Autodesk Inventor part; units mm, degrees
ref_plane "Arbeitsebene1" through (0, 0, 4) normal (0, 0, 1) x (1, 0, 0)
ref_plane "YZ Plane" through (0, 0, 0) normal (1, 0, 0) x (0, 1, 0)
ref_plane "XZ Plane" through (0, 0, 0) normal (0, 1, 0) x (-1, 0, 0)
sketch "Skizze1" plane through (0, 0, 0) normal (0, 0, 1) x (1, 0, 0)
  line L0 (-27, -12) -> (27, -12)
  line L1 (27, -12) -> (27, 12)
  line L2 (27, 12) -> (-27, 12)
  line L3 (-27, 12) -> (-27, -12)
  circle A0 centre (-20, 0) radius 3.05
  circle A1 centre (20, 0) radius 3.05
  arc A2 (-10, 7.5) -> (-10, 2.5) centre (-10, 5) ccw
  arc A3 (10, 2.5) -> (10, 7.5) centre (10, 5) ccw
  line L4 (10, 2.5) -> (-10, 2.5)
  line L5 (10, 7.5) -> (-10, 7.5)
  point P0 (0, 0)
  dimension "d0" = 54
  dimension "d1" = 24
  dimension "d3" = 27
  dimension "d4" = 6.1
  dimension "d5" = 20
  dimension "d6" = 12
  dimension "d7" = 20
  dimension "d8" = 6.1
  dimension "d9" = 12
  dimension "d26" = 4.5
  dimension "d27" = 14.5
  dimension "d28" = 2.5
  dimension "d29" = 20
  dimension "d30" = 10
  dimension "d31" = 12
ref_plane "Arbeitsebene1" through (0, 0, 4) normal (0, 0, 1) x (1, 0, 0)
sketch "Skizze2" plane through (0, 0, 4) normal (0, 0, 1) x (1, 0, 0)
  circle A0 centre (-20, 0) radius 3
  circle A1 centre (20, 0) radius 3
  circle A2 centre (-20, 0) radius 7
  circle A3 centre (-20, 0) radius 3.05
  circle A4 centre (20, 0) radius 3.05
  circle A5 centre (20, 0) radius 7
  point P0 (0, 0)
  dimension "d12" = 6.1
  dimension "d13" = 14
  dimension "d14" = 6.1
  dimension "d15" = 14
extrude "Extrusion2" add sketch "Skizze2" along normal blind 5 contours A2 | A3 | A4 | A5
extrude "Extrusion3" add sketch "Skizze1" along normal blind 4
properties part number "B Montageplatte"
The model under review builds one solid part; all positions refer to its coordinate system, in mm. A direction names the side the tool comes from. Round coordinates to 2 decimals unless told otherwise and drop trailing zeros. Order: outer loops, then holes, each group sorted by start corner. A loop starts at its lowest first (then second) coordinate and runs counter-clockwise, first axis right, second up. Notation, with made-up numbers: (-12.75, 70) -> (26.25, 70) arc R7 ccw to (26.25, 82) -> close; hole circle Ø7 at (12, 21). An arc over 180 degrees is marked (long way). One line per item, written item: value. Start each with the question number.
Q1. Wall thickness on line 1 (X direction, y = 5, z = 0.5); line 2 (X direction, y = 2.25, z = 7.5); line 3 (Y direction, x = 2, z = 0.75): over which ranges is each line inside the solid? List them lowest first.
Q2. Take a section at C-C (z = 5). Write out the cut boundary in (x, y), and give its area (3 significant figures).
Q3. Take a section at A-A (x = -2.5). Write out the cut boundary in (y, z), and give its area (3 significant figures).
Q4. Clearance check with a flat-ended pin moving along its axis: pin 1 Ø5 at (x, y) = (-1, 6) entering from +Z. State where the tip first meets the part, or that it passes through.
Q5. Machinability: for faces 5 (the face through (-17.183, 1.168, 1.972)), 6 (the face through (0, 0, 4)), 7 (the face through (-17, -1, 9)), 8 (the face through (0, 0, 0)), 9 (the face through (12.5, 5.1, 2)), which of the approach directions +Z, -Z, +X, -X, +Y, -Y give a long, thin tool a straight path to every point of the face, cutting with its end or side? Answer none if there is none.
Q6. Take a section at B-B (y = 5). Write out the cut boundary in (x, z).
Q7. Mouldability with a two-part tool opening along X and no side actions: class faces 1 (the face through (-27, 0, 2)), 2 (the face through (23, -1, 9)), 3 (the face through (-23, 0, 6)), 4 (the face through (22.817, 1.168, 1.972)) as released by +X, released by -X, zero draft, split by the parting line, or undercut.
Q8. Take a section at D-D (y = 1.75). Write out the cut boundary in (x, z).
Reported:
1. line 1: x = -27 to -12.5, 12.5 to 27
1. line 2: x = -26.63 to -21.98, -18.02 to -13.37, 13.37 to 18.02, 21.98 to 26.63
1. line 3: y = -12 to 2.5, 7.5 to 12
2. outline: circle Ø14 at (-20, 0); circle Ø14 at (20, 0); hole circle Ø6 at (-20, 0); hole circle Ø6 at (20, 0)
2. area: 251 mm2
3. outline: (-12, 0) -> (2.5, 0) -> (2.5, 4) -> (-12, 4) -> close; (7.5, 0) -> (12, 0) -> (12, 4) -> (7.5, 4) -> close
3. area: 76.0 mm2
4. pin 1: stops at z = 4
5. face 5: -Z
5. face 6: +Z
5. face 7: +Z, +X, -X, +Y, -Y
5. face 8: -Z, +X, -X, +Y, -Y
5. face 9: +Z, -Z
6. outline: (-27, 0) -> (-12.5, 0) -> (-12.5, 4) -> (-15.1, 4) -> (-15.1, 9) -> (-24.9, 9) -> (-24.9, 4) -> (-27, 4) -> close; (12.5, 0) -> (27, 0) -> (27, 4) -> (24.9, 4) -> (24.9, 9) -> (15.1, 9) -> (15.1, 4) -> (12.5, 4) -> close
7. face 1: released by -X
7. face 2: zero draft
7. face 3: undercut
7. face 4: undercut
8. outline: (-27, 0) -> (-22.5, 0) -> (-22.5, 4) -> (-22.44, 4) -> (-22.44, 9) -> (-26.78, 9) -> (-26.78, 4) -> (-27, 4) -> close; (-17.56, 4) -> (-17.5, 4) -> (-17.5, 0) -> (17.5, 0) -> (17.5, 4) -> (17.56, 4) -> (17.56, 9) -> (13.22, 9) -> (13.22, 4) -> (-13.22, 4) -> (-13.22, 9) -> (-17.56, 9) -> close; (22.44, 4) -> (22.5, 4) -> (22.5, 0) -> (27, 0) -> (27, 4) -> (26.78, 4) -> (26.78, 9) -> (22.44, 9) -> close
